CAD build for the part. Positions are in the model's coordinates, mm. A direction names the side the tool comes from. Give positions to 0.01 mm unless a question says otherwise; leave off trailing zeros. Loops run counter-clockwise (first coordinate to the right, second up) from the corner with the lowest first, then second, coordinate; pieces in that order, holes last. Notation, with made-up numbers: M 16.25,6.25 L 22.25,6.25 A21 cw 22.25,33.25 Z; hole C -20,-34.5 d8. An arc over 180 degrees is marked long. Answer as CSV lines item,"result".
```python
from build123d import *

# Parameters (mm, degrees)
F1_DEPTH = 18
F2_R     = 5
F3_R     = 2.25
F4_DEPTH = 8


# Not quite as in the source:
# - a feature names something its author has since deleted; it is built from what else it names


with BuildPart() as f1:
    # F0 (on Front) → F1 (new body)
    with BuildSketch(Plane.XZ):
        with BuildLine():
            ThreePointArc((-64.2237368111, 25.2650516673), (-59.7471801328, 31.1306109239), (-54.3027456241, 26.150402297))
            ThreePointArc((-54.3027456241, 26.150402297), (-56.1661028164, 22.2566288192), (-60.3673343828, 21.2650516673))
            Line((-60.3673343828, 21.2650516673), (-79.3032296173, 21.2650516673))
            Line((-79.3032296173, 21.2650516673), (-79.3043551346, 11.9631245031))
            Line((-79.3043551346, 11.9631245031), (-44.3043551346, 12.150402297))
            Line((-44.3043551346, 12.150402297), (-44.3043551346, 16.150402297))
            ThreePointArc((-44.3043551346, 16.150402297), (-42.5469958217, 20.3930429841), (-38.3043551346, 22.150402297))
            Line((-38.3043551346, 22.150402297), (4.6990865829, 22.150402297))
            ThreePointArc((4.6990865829, 22.150402297), (8.94172727, 20.3930429841), (10.6990865829, 16.150402297))
            Line((10.6990865829, 16.150402297), (10.6990865829, 12.150402297))
            Line((10.6990865829, 12.150402297), (45.6990865829, 12.150402297))
            Line((45.6990865829, 12.150402297), (45.6973702434, 25.2650516673))
            Line((45.6973702434, 25.2650516673), (45.6973702434, 21.2650516673))
            Line((45.6973702434, 21.2650516673), (42.6977375527, 21.2650516673))
            Line((42.6977375527, 21.2650516673), (26.7618431345, 21.2650516673))
            ThreePointArc((26.7618431345, 21.2650516673), (21.803480898, 29.2870451047), (30.6972543759, 26.150402297))
            ThreePointArc((30.6972543759, 26.150402297), (30.6774630028, 25.7059677883), (30.6182455629, 25.2650516673))
            Line((30.6182455629, 25.2650516673), (42.6977375527, 25.2650516673))
            Line((42.6977375527, 25.2650516673), (42.6977375527, 40.3215353384))
            Line((42.6977375527, 40.3215353384), (34.3958526514, 40.3215353384))
            Line((34.3958526514, 40.3215353384), (9.5622779218, 40.3215353384))
            Line((9.5622779218, 40.3215353384), (-22.6043551346, 40.3215353384))
            Line((-22.6043551346, 40.3215353384), (-22.6043551346, 38.3215353384))
            Line((-22.6043551346, 38.3215353384), (-44.3043551346, 38.3215353384))
            Line((-44.3043551346, 38.3215353384), (-66.0043551346, 38.3215353384))
            Line((-66.0043551346, 38.3215353384), (-66.0043551346, 40.3215353384))
            Line((-66.0043551346, 40.3215353384), (-76.3027456241, 40.3215353384))
            Line((-76.3027456241, 40.3215353384), (-76.3027456241, 25.2650516673))
            Line((-76.3027456241, 25.2650516673), (-64.2237368111, 25.2650516673))
        make_face()
    extrude(amount=F1_DEPTH)

    # F2
    f2_edges = [f1.edges().sort_by_distance(p)[0] for p in [
        (-44.304355, -9, 12.150402),
        (10.699087, -9, 12.150402),
    ]]
    fillet(f2_edges, radius=F2_R)

    # F3 (on face) → F4 (cut)
    with BuildSketch(Plane.XY.offset(38.3215353384)):
        with Locations((-30.8043551346, -9)):
            Circle(F3_R)
        with Locations((-57.8043551346, -9)):
            Circle(F3_R)
    extrude(amount=-F4_DEPTH, mode=Mode.SUBTRACT)


solid = f1.part
```
Q1. Cut at C-C (x = -51). Write the cut outline in (y, z), and give its area (3 significant figures).
Solution:
outline,"M -18,12.11 L 0,12.11 L 0,38.32 L -18,38.32 Z"
area,"472 mm²"
Q2. Which spindle directions (+Z, -Z, +X, -X, +Y, -Y) get a long thin tool onto all of the face, cutting with end or side? Do faces 5 (the cylindrical face through (8.7, -8.87, 20.62)), 6 (the flat face through (-70, -9, 21.265)), 7 (the flat face through (-76.303, -9, 33)), 8 (the flat face through (-31, -9, 30.322)). Say none if no direction does.
Solution:
face 5,"-Z, +Y, -Y"
face 6,"-X, +Y, -Y"
face 7,"+Z, -X, +Y, -Y"
face 8,"+Z"
Q3. Cut at B-B (x = -67.5). Write the cut outline in (y, z), and give its area (3 significant figures).
Solution:
outline,"M -18,12.03 L 0,12.03 L 0,21.27 L -18,21.27 Z; M -18,25.27 L 0,25.27 L 0,40.32 L -18,40.32 Z"
area,"437 mm²"
Q4. Cut at A-A (z = 35). Write the cut outline in (x, y), and give its area (3 significant figures).
Solution:
outline,"M -76.3,-18 L 42.7,-18 L 42.7,0 L -76.3,0 Z; hole C -57.8,-9 d4.5; hole C -30.8,-9 d4.5"
area,"2,110 mm²"
Q5. Pin check, flat tips, straight feed: P1, Ø3, axis at x = -44, y = -6.5, coming from the +Z side; P2, Ø5, axis at y = -3.5, z = 29, coming from the -X side; P3, Ø7.5, axis at y = -12.5, z = 30, coming from the +X side; P4, Ø9, axis at x = -59.3, z = 26.15, coming from the -Y side. Stop position of each tip, or through.
Solution:
P1,"stops at z = 38.32"
P2,"stops at x = -76.3"
P3,"stops at x = 42.7"
P4,"passes through"
Q6. Mould opens along Z. For faces 1 (the flat face through (37, -9, 25.265)), 2 (the flat face through (42.698, -9, 33)), 3 (the flat face through (36, -9, 21.265)), 4 (the flat face through (-17, -9, 22.15)) say: released by +Z, released by -Z, zero draft, split by the parting line, or undercut.
Solution:
face 1,"undercut"
face 2,"zero draft"
face 3,"undercut"
face 4,"released by -Z"
Q7. Wall check: line 1 (X direction, y = -14.75, z = 29.5); line 2 (X direction, y = -3.75, z = 27); line 3 (Z direction, x = -22, y = -16). Give the ranges that are in metal, low to high. Write a range as [from, to].
Solution:
line 1,"x = [-76.3, -63.01], [-55.59, 21.99], [29.41, 42.7]"
line 2,"x = [-76.3, -64.23], [-54.38, 20.77], [30.62, 42.7]"
line 3,"z = [22.15, 40.32]"
